Autodesk Inventor part; units mm, degrees
ref_plane "YZ Plane" through (0, 0, 0) normal (1, 0, 0) x (0, 1, 0)
ref_plane "XZ Plane" through (0, 0, 0) normal (0, 1, 0) x (-1, 0, 0)
ref_plane "XY Plane" through (0, 0, 0) normal (0, 0, 1) x (1, 0, 0)
ref_plane "Work Plane1" through (-62.4151, 1.9295, 0) normal (0, 0, 1) x (1, 0, 0)
sketch "Sketch1" plane through (-62.4151, 1.9295, 0) normal (0, 0, 1) x (1, 0, 0)
  line L0 (-5.0959, -1.798) -> (62.2123, -1.798)
  line L1 (62.2123, -1.798) -> (62.2123, 54.509)
  line L2 (62.2123, 54.509) -> (-5.0959, 54.509)
  line L3 (-5.0959, 54.509) -> (-5.0959, -1.798)
  circle A0 centre (-1.5532, 51.0932) radius 1.5
  circle A1 centre (58.9247, 51.1571) radius 1.5
  point P0 (62.4151, -1.9295)
  dimension "d1" = 3
  dimension "d6" = 3
extrude "Extrusion1" add sketch "Sketch1" along normal blind 3
sketch "Sketch3" plane through (-62.4151, 1.9295, 3) normal (0, 0, 1) x (1, 0, 0)
  line L0 (52.7586, 47.7976) -> (2.7586, 47.7976)
  line L1 (2.7586, 47.7976) -> (2.7586, 4.7976)
  line L2 (2.7586, 4.7976) -> (52.7586, 4.7976)
  line L3 (52.7586, 4.7976) -> (52.7586, 47.7976)
  circle A0 centre (5.2586, 7.7976) radius 1
  circle A1 centre (5.2586, 7.7976) radius 1.85
  circle A2 centre (50.2586, 7.7976) radius 1
  circle A3 centre (50.2586, 7.7976) radius 1.85
  circle A4 centre (50.2586, 44.7976) radius 1
  circle A5 centre (50.2586, 44.7976) radius 1.85
  circle A6 centre (5.2586, 44.7976) radius 1
  circle A7 centre (5.2586, 44.7976) radius 1.85
  point P0 (62.4151, -1.9295)
  dimension "d7" = 50
  dimension "d8" = 43
  dimension "d9" = 2
  dimension "d10" = 3.7
  dimension "d11" = 3
  dimension "d12" = 2.5
  dimension "d13" = 2
  dimension "d14" = 3.7
  dimension "d15" = 2
  dimension "d16" = 3.7
  dimension "d17" = 2
  dimension "d18" = 3.7
  dimension "d19" = 3
  dimension "d20" = 2.5
  dimension "d21" = 2.5
  dimension "d22" = 3
  dimension "d23" = 2.5
  dimension "d24" = 3
extrude "Extrusion3" cut sketch "Sketch3" against normal blind 2
sketch "Sketch4" plane through (-62.4151, 1.9295, 1) normal (0, 0, 1) x (1, 0, 0)
  circle A0 centre (50.2586, 7.7976) radius 1
  circle A1 centre (50.2586, 7.7976) radius 1
  circle A2 centre (50.2586, 44.7976) radius 1
  circle A3 centre (50.2586, 44.7976) radius 1
  circle A4 centre (5.2586, 44.7976) radius 1
  circle A5 centre (5.2586, 44.7976) radius 1
  circle A6 centre (5.2586, 7.7976) radius 1
  circle A7 centre (5.2586, 7.7976) radius 1
  point P0 (62.4151, -1.9295)
extrude "Extrusion4" cut sketch "Sketch4" against normal through all
sketch "Sketch5" plane through (-62.4151, 1.9295, 3) normal (0, 0, 1) x (1, 0, 0)
  line L0 (-5.0959, -1.798) -> (62.2123, -1.798)
  line L1 (55.2123, -1.798) -> (1.9041, -1.798)
  line L2 (1.9041, -1.798) -> (1.9041, 2.202)
  line L3 (1.9041, 2.202) -> (55.2123, 2.202)
  line L4 (55.2123, 2.202) -> (55.2123, -1.798)
  line L5 (62.2123, 54.509) -> (-5.0959, 54.509)
  line L6 (6.9041, 54.509) -> (50.2123, 54.509)
  line L7 (50.2123, 54.509) -> (50.2123, 50.509)
  line L8 (50.2123, 50.509) -> (6.9041, 50.509)
  line L9 (6.9041, 50.509) -> (6.9041, 54.509)
  line L10 (62.2123, -1.798) -> (62.2123, 54.509)
  line L11 (-5.0959, 54.509) -> (-5.0959, -1.798)
  point P0 (62.4151, -1.9295)
  point P1 (50.2123, 52.509)
  point P2 (6.9041, 52.509)
  point P3 (1.9041, 0.202)
  point P4 (55.2123, 0.202)
  dimension "d29" = 4
  dimension "d30" = 4
  dimension "d31" = 12
  dimension "d32" = 12
  dimension "d33" = 7
  dimension "d34" = 7
extrude "Extrusion5" cut sketch "Sketch5" against normal through all contours L2 L3 L4 L0 | L5 L7 L8 L9
properties part number "RelayTray"
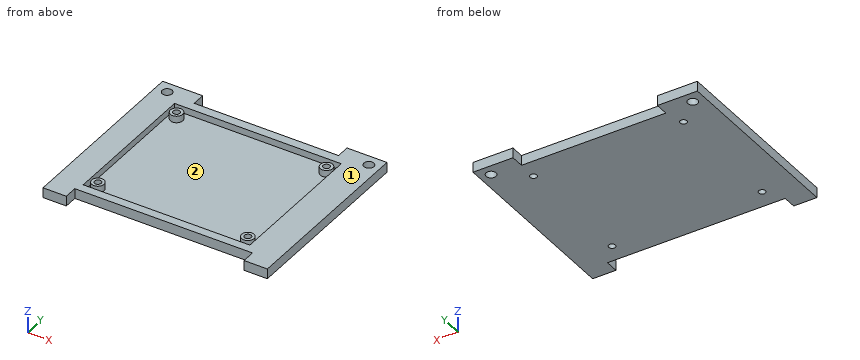
Work out the finished part from the listing and answer in its coordinate system (mm). Face numbers are marked on the shaded views. Give positions to 0.01 mm unless a question says otherwise; leave off trailing zeros. Order: outer loops, then holes, each group sorted by start corner. A loop starts at its lowest first (then second) coordinate and runs counter-clockwise, first axis right, second up. Notation, with made-up numbers: (35.5, 14.25) -> (84.5, 14.25) arc R28 ccw to (84.5, 37.25) -> close; hole circle Ø6 at (-26.5, 29.5). An arc over 180 degrees is marked (long way). One line per item, written item: value.
Item 1: Find section B-B, the plane y = 43.5. Give the vertices of the cut face in (x, z), plus the area to 3 significant figures.
Answer sheet:
outline: (-67.51, 0) -> (-0.2, 0) -> (-0.2, 3) -> (-9.66, 3) -> (-9.66, 1) -> (-59.66, 1) -> (-59.66, 3) -> (-67.51, 3) -> close
area: 102 mm²
Item 2: Flat-ended cylindrical pins translate along their axes: P1, Ø1.5, axis at x = -38.5, z = 1, coming from the +Y side; P2, Ø1, axis at x = -25.5, z = 2, coming from the -Y side; P3, Ø4, axis at x = -3.49, y = 53.09, coming from the -Z side; P4, Ø4, axis at x = -47, y = 10.5, coming from the +Z side. Find the tip coordinate at first contact, or state that the pin passes through.
Answer sheet:
P1: y = 52.44
P2: y = 4.13
P3: z = 0
P4: z = 1
Item 3: Find section C-C, the plane x = -26. Give the vertices of the cut face in (y, z).
Answer sheet:
outline: (4.13, 0) -> (52.44, 0) -> (52.44, 3) -> (49.73, 3) -> (49.73, 1) -> (6.73, 1) -> (6.73, 3) -> (4.13, 3) -> close
Item 4: Find section A-A, the plane z = 1.5. State how many separate pieces and enclosed holes the cut face has, plus the area to 3 significant figures.
Answer sheet:
separate pieces: 5
enclosed holes: 7
area: 1,270 mm²
Item 5: Straight lines are drawn through the part: probe 1 along X at (y, z) = (4, 1.1); probe 2 along X at (y, z) = (37, 2.95); probe 3 along Y at (x, z) = (-24.5, 2.55). For each, find the intervals that lie inside material, in ascending order.
Answer sheet:
probe 1: -67.51 to -60.51, -7.2 to -0.2
probe 2: -67.51 to -59.66, -9.66 to -0.2
probe 3: 4.13 to 6.73, 49.73 to 52.44
Item 6: Determine the mould class of the marked faces 1 and 2 for opening direction Y: released by +Y, released by -Y, zero draft, split by the parting line, or undercut.
Answer sheet:
face 1: zero draft
face 2: undercut
